from build123d import *

# Parameters (mm, degrees)
SKETCH_1_W      = 100
SKETCH_1_H      = 100
SKETCH_1_R      = 20
EXTRUDE_1_DEPTH = 100
FILLET_1_R      = 5
FILLET_2_R      = 5


with BuildPart() as part:
    # 草图1 → 凸台-拉伸1 (new body)
    with BuildSketch(Plane.XY):
        Rectangle(SKETCH_1_W, SKETCH_1_H)
        Circle(SKETCH_1_R, mode=Mode.SUBTRACT)
    extrude(amount=EXTRUDE_1_DEPTH)

    # 圆角1
    fillet_1_edges = [part.edges().sort_by_distance(p)[0] for p in [
        (-50, 0, 100),
        (0, -50, 100),
        (50, 0, 100),
        (0, -50, 0),
        (-50, 0, 0),
        (0, 50, 0),
        (50, 0, 0),
        (50, -50, 50),
        (-50, -50, 50),
        (-50, 50, 50),
        (50, 50, 50),
        (0, 50, 100),
    ]]
    fillet(fillet_1_edges, radius=FILLET_1_R)

    # 圆角2
    fillet_2_edges = [part.edges().sort_by_distance(p)[0] for p in [
        (-20, 0, 0),
        (-20, 0, 100),
    ]]
    fillet(fillet_2_edges, radius=FILLET_2_R)


solid = part.part
Can you work these out from the model? Positions are in its coordinate system, mm. Give positions to 0.01 mm unless a question says otherwise; leave off trailing zeros. Write each loop counter-clockwise with the first axis right and the second up, starting at its lowest first coordinate (ties: lowest second). Pieces come first, ordered by that corner, then holes. Notation, with made-up numbers: M 17.25,75 L 33.25,75 A25 cw 33.25,97 Z; hole C -16.5,-17.5 d6. An arc over 180 degrees is marked long. Answer in a Markdown table with one row per item. Add a question column.
Item 1: Imagine slicing it at B-B, the plane z = 12.5. Write out the boundary of the cut face in (x, y), plus the area to 3 significant figures.
Item 2: Please list where these lines run through material, in increasing order: L1, parallel to Y at x = 0, z = 42; L2, parallel to X at y = -9.5, z = 74.5; L3, parallel to Y at x = -18, z = 34.5.
Item 3: Imagine slicing it at A-A, the plane x = 0. Write out the boundary of the cut face in (y, z), plus the area to 3 significant figures.
Item 4: We'd pull the mould along Z, two halves only. Please class faces 1 (the cylindrical face through (1, -49, 98)), 2 (the flat face through (-1, 50, 49)), 3 (the cylindrical face through (-49, 1, 2)): released by +Z, released by -Z, zero draft, split by the parting line, or undercut.
Evaluation:
| question | item | result |
|---|---|---|
| 1 | outline | M -50,-45 A5 ccw -45,-50 L 45,-50 A5 ccw 50,-45 L 50,45 A5 ccw 45,50 L -45,50 A5 ccw -50,45 Z; hole C 0,0 d40 |
| 1 | area | 8,720 mm² |
| 2 | L1 | y = -50 to -20, 20 to 50 |
| 2 | L2 | x = -50 to -17.6, 17.6 to 50 |
| 2 | L3 | y = -50 to -8.72, 8.72 to 50 |
| 3 | outline | M -50,5 A5 ccw -45,0 L -25,0 A5 ccw -20,5 L -20,95 A5 ccw -25,100 L -45,100 A5 ccw -50,95 Z; M 20,5 A5 ccw 25,0 L 45,0 A5 ccw 50,5 L 50,95 A5 ccw 45,100 L 25,100 A5 ccw 20,95 Z |
| 3 | area | 5,960 mm² |
| 4 | face 1 | released by +Z |
| 4 | face 2 | zero draft |
| 4 | face 3 | released by -Z |
